from build123d import *

# Parameters (mm, degrees)
SKETCH1_W           = 28
SKETCH1_H           = 9
SKETCH1_R           = 1.5
SKETCH1_W_2         = 3
SKETCH1_H_2         = 17.5
BOSS_EXTRUDE1_DEPTH = 2


with BuildPart() as part:
    # Sketch1 → Boss-Extrude1 (new body)
    with BuildSketch(Plane.XY):
        with Locations((14, 4.5)):
            Rectangle(SKETCH1_W, SKETCH1_H)
        with Locations((5, 4.75)):
            Circle(SKETCH1_R, mode=Mode.SUBTRACT)
        with Locations((23, 4.75)):
            Circle(SKETCH1_R, mode=Mode.SUBTRACT)
        with Locations((14, -8.75)):
            Rectangle(SKETCH1_W_2, SKETCH1_H_2)
    extrude(amount=BOSS_EXTRUDE1_DEPTH)


solid = part.part
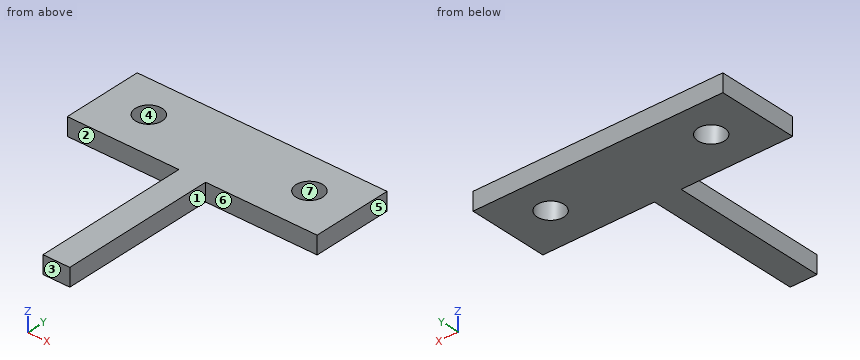
Could you check a few things on this model? Use its own coordinates, in mm. Face numbers are marked on the shaded views. A direction names the side the tool comes from. Coordinates: 2 decimals unless noted, no trailing zeros. Order: outer loops, then holes, each group sorted by start corner. A loop starts at its lowest first (then second) coordinate and runs counter-clockwise, first axis right, second up. Notation, with made-up numbers: (-8, 18.25) - (37, 18.25) arc R29 cw to (37, 52.25) - close; hole circle Ø10 at (-23, -18). An arc over 180 degrees is marked (long way). Answer in a Markdown table with one row per item. Add a question column.
(1) If we mould it in two halves opening along Y, with no side actions, what happens to the marked faces 4, 5, 6 and 7? For each: released by +Y, released by -Y, zero draft, split by the parting line, or undercut.
(2) On a 3-axis mill with a long thin cutter (end or side, diameter ignored), from which of +Z, -Z, +X, -X, +Y, -Y can I reach the whole of each face in a straight line? I mean the marked faces 1, 2 and 3. Say none if no direction works.
(3) I need wall thicknesses on L1, parallel to X at y = 5, z = 1.75; L2, parallel to X at y = 3.75, z = 0.15; L3, parallel to Y at x = 5, z = 1.5. Which ranges of each line are inside material? Lowest first, please.
(4) If we section it at A-A, the plane y = 4.75: Please give me the cut outline in (x, z).
(5) If we section it at D-D, the plane y = -6.5: Please give me the cut outline in (x, z), then the cut area to 3 significant figures.
(6) If we section it at C-C, the plane z = 0.3: Please give me the cut outline in (x, y), then the cut area to 3 significant figures.
(7) Will these pins go through, and if not, where does the flat tip stop? pin 1 (6 mm diameter, centred on x = 8.5, y = -13.5, fed in from -Z); pin 2 (1 mm diameter, centred on x = 21.5, z = 1.5, fed in from -Y).
(8) If we section it at B-B, the plane x = 5: Please give me the cut outline in (y, z).
Results are:
| question | item | result |
|---|---|---|
| 1 | face 4 | undercut |
| 1 | face 5 | zero draft |
| 1 | face 6 | released by -Y |
| 1 | face 7 | undercut |
| 2 | face 1 | +Z, -Z, +X, -Y |
| 2 | face 2 | +Z, -Z, -X, -Y |
| 2 | face 3 | +Z, -Z, +X, -X, -Y |
| 3 | L1 | x = 0 to 3.52, 6.48 to 21.52, 24.48 to 28 |
| 3 | L2 | x = 0 to 3.88, 6.12 to 21.88, 24.12 to 28 |
| 3 | L3 | y = 0 to 3.25, 6.25 to 9 |
| 4 | outline | (0, 0) - (3.5, 0) - (3.5, 2) - (0, 2) - close; (6.5, 0) - (21.5, 0) - (21.5, 2) - (6.5, 2) - close; (24.5, 0) - (28, 0) - (28, 2) - (24.5, 2) - close |
| 5 | outline | (12.5, 0) - (15.5, 0) - (15.5, 2) - (12.5, 2) - close |
| 5 | area | 6.00 mm2 |
| 6 | outline | (0, 0) - (12.5, 0) - (12.5, -17.5) - (15.5, -17.5) - (15.5, 0) - (28, 0) - (28, 9) - (0, 9) - close; hole circle Ø3 at (5, 4.75); hole circle Ø3 at (23, 4.75) |
| 6 | area | 290 mm2 |
| 7 | pin 1 | passes through |
| 7 | pin 2 | stops at y = 0 |
| 8 | outline | (0, 0) - (3.25, 0) - (3.25, 2) - (0, 2) - close; (6.25, 0) - (9, 0) - (9, 2) - (6.25, 2) - close |
